Design review of the part shown in the three views and the two pictorial views. Dimensions are in mm from the part's minimum x, y and z. Round coordinates to 2 decimals unless told otherwise and drop trailing zeros. Loops run counter-clockwise (first coordinate to the right, second up) from the corner with the lowest first, then second, coordinate; pieces in that order, holes last. Notation, with made-up numbers: M 23.5,39 L 65.5,39 A24 cw 65.5,50 Z; hole C 80,-36.75 d2. An arc over 180 degrees is marked long. One line per question, with ' | ' between items.
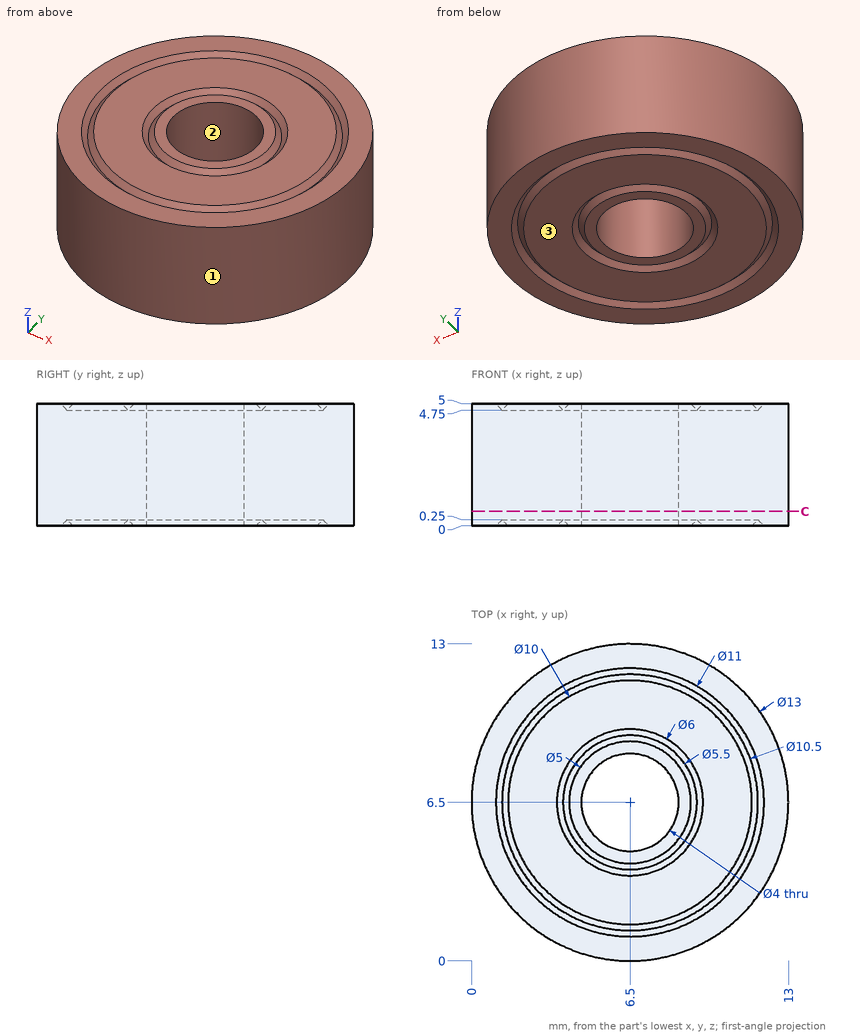
1) For line 1 (Y direction, x = 6.5, z = 3.75); line 2 (Y direction, x = 5.25, z = 2.45); line 3 (Y direction, x = 0.5, z = 2.25), list the stretches that pass through material, from the lowest coordinate up.
Output values:
line 1: y = 0 to 4.5, 8.5 to 13 | line 2: y = 0.12 to 4.94, 8.06 to 12.88 | line 3: y = 4 to 9
2) Insertion check: P1, Ø2.5, axis at x = 6.5, y = 6.5, coming from the +Z side; P2, Ø1, axis at x = 3, z = 1.5, coming from the -Y side; P3, Ø1.5, axis at y = 2.5, z = 3, coming from the -X side. Each pin has a flat end and moves straight along its axis. Give the tip position at first contact, or say it passes through.
Output values:
P1: passes through | P2: stops at y = 0.73 | P3: stops at x = 0.87
3) Mouldability with a two-part tool opening along X and no side actions: class the marked faces 1, 2 and 3 as +X half, -X half, draft (parallel to the pull), parting line (faces both ways), or undercut.
Output values:
face 1: parting line | face 2: undercut | face 3: draft
4) Add section C-C on z = 0.6. State the section outline as (x, y) points.
Output values:
outline: C 6.5,6.5 d13; hole C 6.5,6.5 d4
